Read the model definition and answer for the solid it produces. Units are mm, in the model's axes. Coordinates: 2 decimals unless noted, no trailing zeros. Loops run counter-clockwise (first coordinate to the right, second up) from the corner with the lowest first, then second, coordinate; pieces in that order, holes last. Notation, with made-up numbers: (76.25, 80.5) -> (132.25, 80.5) arc R14 cw to (132.25, 101.5) -> close; hole circle Ø6 at (79.5, 31.5). An arc over 180 degrees is marked (long way). Answer as a JSON object with one key per item and string values. Group by question number.
1) Section B-B, the plane z = -3.2 is taken. Count the separate pieces of the cut face and the enclosed holes in it, plus the area to 3 significant figures.
2) Flat-ended cylindrical pins translate along their axes: P1, Ø2, axis at x = -20, z = -2.5, coming from the -Y side; P2, Ø8, axis at x = -86.868, y = -16.51, coming from the +Z side. Find the tip coordinate at first contact, or state that the pin passes through.
3) Consider probe 1 along X at (y, z) = (-36, -3.2); probe 2 along Y at (x, z) = (-55, -0.15); probe 3 along X at (y, z) = (29, -2.55). Determine where each line is inside the solid, lowest interval first. Write a range as [from, to].
4) Determine the mould class of faces 1 (the face through (-3, 36, 0)), 2 (the face through (-43.41, 52.95, -2.5)) for opening direction Y: released by +Y, released by -Y, zero draft, split by the parting line, or undercut.
5) Section A-A, the plane x = -160 is taken. Give the vertices of the cut face in (y, z), plus the area to 3 significant figures.
from build123d import *

# Parameters (mm, degrees)
SKETCH2_R           = 3.048
BOSS_EXTRUDE1_DEPTH = 5.07492
CUT_EXTRUDE11_DEPTH = 210.646067011
SKETCH3_R           = 6.35
SKETCH3_R_2         = 2.032
CUT_EXTRUDE12_DEPTH = 210.646067011
SKETCH5_R           = 1.4732
CUT_EXTRUDE13_DEPTH = 210.646067011
SKETCH7_R           = 1.905
CUT_EXTRUDE14_DEPTH = 210.646067011
SKETCH8_R           = 3.175
CUT_EXTRUDE15_DEPTH = 210.646067011


with BuildPart() as part:
    # Sketch2 → Boss-Extrude1 (new body)
    with BuildSketch(Plane.XY):
        with BuildLine():
            Line((-186.69, -31.75), (-144.826640797, -31.75))
            ThreePointArc((-144.826640797, -31.75), (-123.19, -59.055), (-101.553359203, -31.75))
            Line((-101.553359203, -31.75), (101.553359203, -31.75))
            ThreePointArc((101.553359203, -31.75), (123.19, -59.055), (144.826640797, -31.75))
            Line((144.826640797, -31.75), (186.69, -31.75))
            Line((186.69, -31.75), (186.69, 95.25))
            Line((186.69, 95.25), (-186.69, 95.25))
            Line((-186.69, 95.25), (-186.69, -31.75))
        make_face()
        with Locations((-86.868, -16.51)):
            Circle(SKETCH2_R, mode=Mode.SUBTRACT)
        with Locations((86.868, -16.51)):
            Circle(SKETCH2_R, mode=Mode.SUBTRACT)
        with Locations((123.19, 76.2)):
            Circle(SKETCH2_R, mode=Mode.SUBTRACT)
        with Locations((-123.19, 76.2)):
            Circle(SKETCH2_R, mode=Mode.SUBTRACT)
    extrude(amount=-BOSS_EXTRUDE1_DEPTH)

    # Sketch2_4 → Cut-Extrude11 (cut, through all)
    with BuildSketch(Plane.XY):
        with BuildLine():
            ThreePointArc((-119.486801079, -31.75), (-123.19, -30.5435), (-126.893198921, -31.75))
            Line((-126.893198921, -31.75), (-119.486801079, -31.75))
        make_face()
        with BuildLine():
            Line((-119.486801079, -31.75), (-126.893198921, -31.75))
            ThreePointArc((-126.893198921, -31.75), (-126.039554547, -42.433581099), (-116.9035, -36.83))
            ThreePointArc((-116.9035, -36.83), (-117.586418901, -33.980445453), (-119.486801079, -31.75))
        make_face()
        with BuildLine():
            ThreePointArc((126.893198921, -31.75), (123.19, -30.5435), (119.486801079, -31.75))
            Line((119.486801079, -31.75), (126.893198921, -31.75))
        make_face()
        with BuildLine():
            Line((126.893198921, -31.75), (119.486801079, -31.75))
            ThreePointArc((119.486801079, -31.75), (120.340445453, -42.433581099), (129.4765, -36.83))
            ThreePointArc((129.4765, -36.83), (128.793581099, -33.980445453), (126.893198921, -31.75))
        make_face()
    extrude(amount=-CUT_EXTRUDE11_DEPTH, mode=Mode.SUBTRACT)

    # Sketch3 → Cut-Extrude12 (cut, through all)
    with BuildSketch(Plane.XY):
        with Locations((-37.066912964, 52.668292248)):
            Circle(SKETCH3_R)
        with Locations((-19.540912964, 52.668292248)):
            Circle(SKETCH3_R_2)
        with Locations((41.776586977, -2.799378671)):
            Circle(SKETCH3_R)
        with Locations((59.302586977, -2.799378671)):
            Circle(SKETCH3_R_2)
        with Locations((41.776586977, 14.726621329)):
            Circle(SKETCH3_R_2)
        with Locations((24.250586977, -2.799378671)):
            Circle(SKETCH3_R_2)
        with Locations((-37.066912964, 70.194292248)):
            Circle(SKETCH3_R_2)
        with Locations((-54.592912964, 52.668292248)):
            Circle(SKETCH3_R_2)
        with Locations((-37.066912964, 35.142292248)):
            Circle(SKETCH3_R_2)
        with Locations((41.776586977, -20.325378671)):
            Circle(SKETCH3_R_2)
    extrude(amount=-CUT_EXTRUDE12_DEPTH, mode=Mode.SUBTRACT)

    # Sketch5 → Cut-Extrude13 (cut, through all)
    with BuildSketch(Plane.XY):
        with Locations((-57.204064287, 29.45032738)):
            Circle(SKETCH5_R)
        with Locations((-16.929761641, 29.45032738)):
            Circle(SKETCH5_R)
        with Locations((-67.25069254, 46.878801212)):
            Circle(SKETCH5_R)
        with Locations((-6.883133387, 46.878801212)):
            Circle(SKETCH5_R)
        with Locations((21.639435654, -26.017343538)):
            Circle(SKETCH5_R)
        with Locations((61.9137383, -26.017343538)):
            Circle(SKETCH5_R)
        with Locations((11.5928074, -8.588869707)):
            Circle(SKETCH5_R)
        with Locations((71.960366554, -8.588869707)):
            Circle(SKETCH5_R)
    extrude(amount=-CUT_EXTRUDE13_DEPTH, mode=Mode.SUBTRACT)

    # Sketch7 → Cut-Extrude14 (cut, through all)
    with BuildSketch(Plane.XY):
        with Locations((131.572, -19.05)):
            Circle(SKETCH7_R)
        with Locations((114.808, -19.05)):
            Circle(SKETCH7_R)
        with Locations((-123.19, -49.022)):
            Circle(SKETCH7_R)
        with Locations((-131.572, -19.05)):
            Circle(SKETCH7_R)
        with Locations((-114.808, -19.05)):
            Circle(SKETCH7_R)
        with Locations((123.19, -49.022)):
            Circle(SKETCH7_R)
    extrude(amount=-CUT_EXTRUDE14_DEPTH, mode=Mode.SUBTRACT)

    # Sketch8 → Cut-Extrude15 (cut, through all)
    with BuildSketch(Plane.XY):
        with Locations((0, -23.114)):
            Circle(SKETCH8_R)
    extrude(amount=-CUT_EXTRUDE15_DEPTH, mode=Mode.SUBTRACT)


solid = part.part
Determined:
{
 "1": {"separate pieces": "1", "enclosed holes": "31", "area": "48,500 mm²"},
 "2": {"P1": "y = -31.75", "P2": "z = 0"},
 "3": {"probe 1": "[-145.4, -129.42], [-116.96, -100.98], [100.98, 116.96], [129.42, 145.4]", "probe 2": "[-31.75, 50.68], [54.66, 95.25]", "probe 3": "[-186.69, -58.61], [-55.8, -18.33], [-15.53, 186.69]"},
 "4": {"face 1": "zero draft", "face 2": "undercut"},
 "5": {"outline": "(-31.75, -5.07) -> (95.25, -5.07) -> (95.25, 0) -> (-31.75, 0) -> close", "area": "645 mm²"}
}
